Answer from the drawing. Dimensions are ordinates in mm from the lowest x, y and z of the part. Coordinates: 2 decimals unless noted, no trailing zeros. Write each loop counter-clockwise with the first axis right and the second up, starting at its lowest first coordinate (ties: lowest second). Pieces come first, ordered by that corner, then holes. Notation, with made-up numbers: (9, 29) -> (19, 29) arc R15 cw to (19, 58) -> close; hole circle Ø3 at (55.25, 59). An arc over 180 degrees is marked (long way). Return JSON: item names as keys, results as strings.
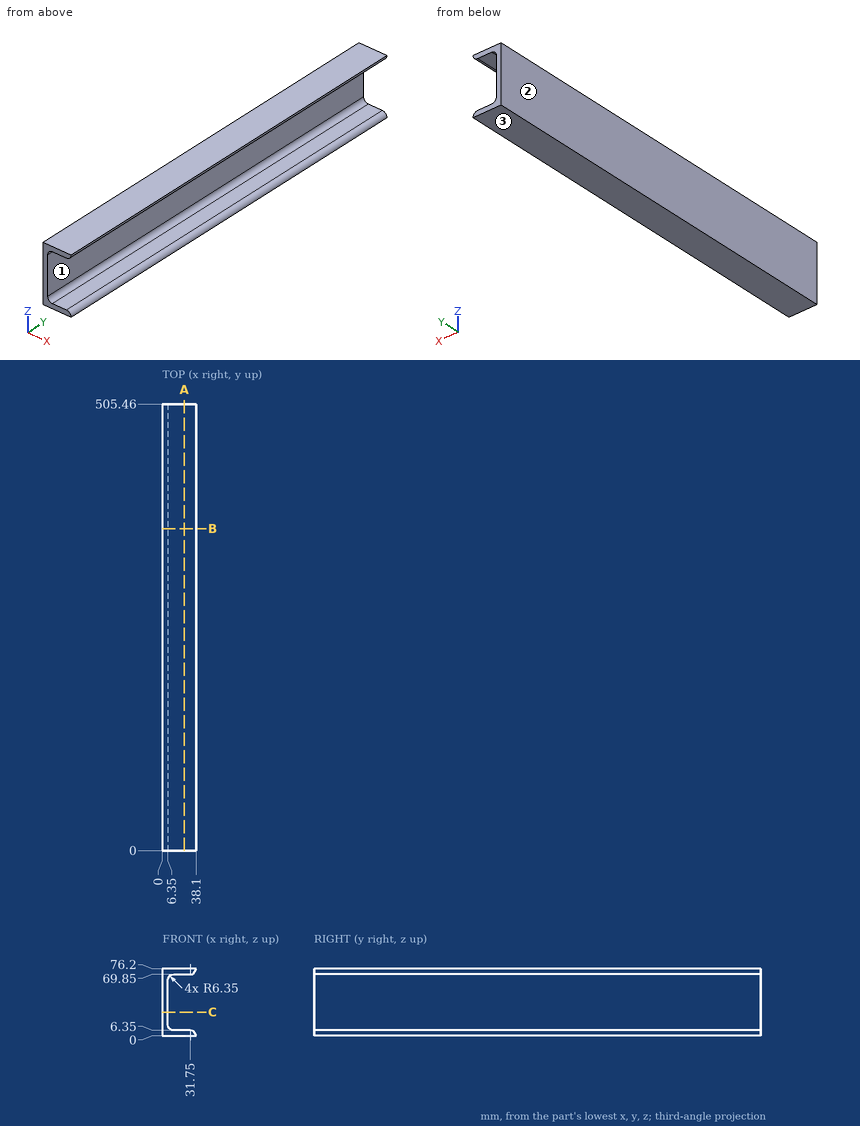
1. For a pull along Z with two mould halves and no side action, classify the marked faces 1, 2 and 3 as +Z half, -Z half, draft (parallel to the pull), parting line (faces both ways), or undercut.
Taken from the geometry:
{"face 1": "undercut", "face 2": "draft", "face 3": "-Z half"}
2. The part is cut by section C-C (z = 27). Determine the outline of the cut face in (x, y).
Taken from the geometry:
{"outline": "(0, 0) -> (6.35, 0) -> (6.35, 505.46) -> (0, 505.46) -> close"}
3. The part is cut by section A-A (x = 25). Determine the outline of the cut face in (y, z), then the cut area to 3 significant figures.
Taken from the geometry:
{"outline": "(0, 0) -> (505.46, 0) -> (505.46, 6.35) -> (0, 6.35) -> close; (0, 69.85) -> (505.46, 69.85) -> (505.46, 76.2) -> (0, 76.2) -> close", "area": "6,420 mm2"}
4. The part is cut by section B-B (y = 364.5). Determine the outline of the cut face in (x, z), then the cut area to 3 significant figures.
Taken from the geometry:
{"outline": "(0, 0) -> (38.1, 0) arc R6.35 ccw to (31.75, 6.35) -> (12.7, 6.35) arc R6.35 cw to (6.35, 12.7) -> (6.35, 63.5) arc R6.35 cw to (12.7, 69.85) -> (31.75, 69.85) arc R6.35 ccw to (38.1, 76.2) -> (0, 76.2) -> close", "area": "887 mm2"}
5. Consider L1, parallel to Z at x = 21, y = 217; L2, parallel to X at y = 229, z = 62; L3, parallel to Z at x = 10, y = 399. Determine where each line is inside the solid, lowest interval first.
Taken from the geometry:
{"L1": "z = 0 to 6.35, 69.85 to 76.2", "L2": "x = 0 to 6.35", "L3": "z = 0 to 6.95, 69.25 to 76.2"}
